Read the model definition and answer for the solid it produces. Units are mm, in the model's axes. A direction names the side the tool comes from. Coordinates: 2 decimals unless noted, no trailing zeros. Loops run counter-clockwise (first coordinate to the right, second up) from the corner with the lowest first, then second, coordinate; pieces in that order, holes last. Notation, with made-up numbers: (-25, -14) -> (-8, -14) arc R30 ccw to (-8, 17) -> close; hole circle Ø9 at (-2.5, 18). An arc over 180 degrees is marked (long way). Answer in a Markdown table with one row per item.
```python
from build123d import *

# Parameters (mm, degrees)
SKETCH2_R          = 1.5875
CUT_EXTRUDE1_DEPTH = 26.48585


with BuildPart() as part:
    # Sketch1 → Revolve1 (revolve)
    with BuildSketch(Plane.XY):
        with BuildLine():
            Line((-0.919083697, 24.909383697), (-0.52705, 24.51735))
            Line((-0.52705, 24.51735), (0, 24.51735))
            Line((0, 24.51735), (1.0541, 25.57145))
            Line((1.0541, 25.57145), (67.9577, 25.57145))
            Line((67.9577, 25.57145), (69.0118, 24.51735))
            Line((69.0118, 24.51735), (69.53885, 24.51735))
            Line((69.53885, 24.51735), (69.930883697, 24.909383697))
            ThreePointArc((69.930883697, 24.909383697), (69.968081136, 24.999186258), (69.930883697, 25.088988819))
            Line((69.930883697, 25.088988819), (68.842761258, 26.177111258))
            ThreePointArc((68.842761258, 26.177111258), (68.500786606, 26.405611415), (68.0974, 26.48585))
            Line((68.0974, 26.48585), (0.9144, 26.48585))
            ThreePointArc((0.9144, 26.48585), (0.511013394, 26.405611415), (0.169038742, 26.177111258))
            Line((0.169038742, 26.177111258), (-0.919083697, 25.088988819))
            ThreePointArc((-0.919083697, 25.088988819), (-0.956281136, 24.999186258), (-0.919083697, 24.909383697))
        make_face()
    revolve(axis=Axis((69.0118, 0, 0), (-1, 0, 0)))

    # Sketch2 → Cut-Extrude1 (cut)
    with BuildSketch(Plane.XY):
        with Locations((57.3659, 0)):
            Circle(SKETCH2_R)
    extrude(amount=CUT_EXTRUDE1_DEPTH, mode=Mode.SUBTRACT)


solid = part.part
```
1. Find the intervals of material crossed by probe 1 along Y at (x, z) = (39.5, 0); probe 2 along Z at (x, y) = (60, 6.5), in increasing order.
A:
| item | result |
|---|---|
| probe 1 | y = -26.49 to -25.57, 25.57 to 26.49 |
| probe 2 | z = -25.68 to -24.73, 24.73 to 25.68 |
2. A cutting plane is placed at C-C on x = 3. Give the vertices of the cut face in (y, z), and give its area (3 significant figures).
A:
| item | result |
|---|---|
| outline | circle Ø52.97 at (0, 0); hole circle Ø51.14 at (0, 0) |
| area | 150 mm2 |
3. A cutting plane is placed at B-B on z = 0. Give the vertices of the cut face in (x, y), and give its area (3 significant figures).
A:
| item | result |
|---|---|
| outline | (-0.92, -25.09) -> (0.17, -26.18) arc R1.05 ccw to (0.91, -26.49) -> (68.1, -26.49) arc R1.05 ccw to (68.84, -26.18) -> (69.93, -25.09) arc R0.13 ccw to (69.93, -24.91) -> (69.54, -24.52) -> (69.01, -24.52) -> (67.96, -25.57) -> (1.05, -25.57) -> (0, -24.52) -> (-0.53, -24.52) -> (-0.92, -24.91) arc R0.13 ccw to start; (-0.92, 24.91) -> (-0.53, 24.52) -> (0, 24.52) -> (1.05, 25.57) -> (67.96, 25.57) -> (69.01, 24.52) -> (69.54, 24.52) -> (69.93, 24.91) arc R0.13 ccw to (69.93, 25.09) -> (68.84, 26.18) arc R1.05 ccw to (68.1, 26.49) -> (0.91, 26.49) arc R1.05 ccw to (0.17, 26.18) -> (-0.92, 25.09) arc R0.13 ccw to start |
| area | 131 mm2 |
4. The mould has two halves that part along X. Classify faces 1 (the cylindrical face through (-0.26, -18.07, -16.57)), 2 (the cylindrical face through (58.88, 0.48, 26)): pulls with the +X half, pulls with the -X half, needs draft (parallel to the pull), parting line crosses it, or undercut.
A:
| item | result |
|---|---|
| face 1 | needs draft |
| face 2 | undercut |
5. A tool of negligible diameter and unlimited length cuts with its end or side. For faces 3 (the cylindrical face through (34.04, 25.26, -7.96)), 4 (the cylindrical face through (34.974, 23.622, 9.794)), from which of +Z, -Z, +X, -X, +Y, -Y can it reach the whole face along a straight path? Write none if from no direction.
A:
| item | result |
|---|---|
| face 3 | +X, -X |
| face 4 | none |
6. Given pin 1 Ø4 at (y, z) = (16, 17.5) entering from -X; pin 2 Ø4 at (x, y) = (36.5, -10.5) entering from -Z; pin 3 Ø6 at (x, z) = (10, 18.5) entering from -Y; pin 4 Ø10 at (x, z) = (25, 12.5) entering from +Y, each flat-ended and moving along its own axis, determine where each tip first touches the part or whether it passes through.
A:
| item | result |
|---|---|
| pin 1 | stops at x = -0.96 |
| pin 2 | stops at z = -25.08 |
| pin 3 | stops at y = -21.48 |
| pin 4 | stops at y = 25.4 |
7. A cutting plane is placed at A-A on y = 0. Count the separate pieces of the cut face and the enclosed holes in it, and give its area (3 significant figures).
A:
| item | result |
|---|---|
| separate pieces | 3 |
| enclosed holes | 0 |
| area | 128 mm2 |
